The listing builds one solid part. Answer for the finished solid, in the listing's coordinates (mm). Give positions to 0.01 mm unless a question says otherwise; leave off trailing zeros. Order: outer loops, then holes, each group sorted by start corner. A loop starts at its lowest first (then second) coordinate and runs counter-clockwise, first axis right, second up. Notation, with made-up numbers: (25.25, -14) - (56.25, -14) arc R13 cw to (56.25, 8) - close; hole circle Ø10 at (-18, 22). An arc over 180 degrees is marked (long way). Use CSV: the item, a comma, the result in double quotes.
```python
from build123d import *

# Parameters (mm, degrees)
F0_W     = 178
F0_H     = 132
F0_R     = 1.6
F0_R_2   = 1.85
F0_R_3   = 4
F1_DEPTH = 25


with BuildPart() as f1:
    # F0 (on Front) → F1 (new body)
    with BuildSketch(Plane.XZ):
        with Locations((0, -66)):
            Rectangle(F0_W, F0_H)
        with Locations((-33, -112)):
            Circle(F0_R, mode=Mode.SUBTRACT)
        with Locations((-78.656854, -85.656854)):
            Circle(F0_R_2, mode=Mode.SUBTRACT)
        with Locations((-73, -88)):
            Circle(F0_R_2, mode=Mode.SUBTRACT)
        with Locations((-67.343146, -85.656854)):
            Circle(F0_R_2, mode=Mode.SUBTRACT)
        with Locations((-81, -80)):
            Circle(F0_R_2, mode=Mode.SUBTRACT)
        with Locations((-78.656854, -74.343146)):
            Circle(F0_R_2, mode=Mode.SUBTRACT)
        with Locations((-73, -80)):
            Circle(F0_R_3, mode=Mode.SUBTRACT)
        with Locations((-67.343146, -74.343146)):
            Circle(F0_R_2, mode=Mode.SUBTRACT)
        with Locations((-73, -72)):
            Circle(F0_R_2, mode=Mode.SUBTRACT)
        with Locations((-65, -80)):
            Circle(F0_R_2, mode=Mode.SUBTRACT)
        with Locations((19.5, -108)):
            Circle(F0_R, mode=Mode.SUBTRACT)
        with Locations((19.5, -80)):
            Circle(F0_R, mode=Mode.SUBTRACT)
        with Locations((65.343146, -85.656854)):
            Circle(F0_R_2, mode=Mode.SUBTRACT)
        with Locations((71, -88)):
            Circle(F0_R_2, mode=Mode.SUBTRACT)
        with Locations((76.656854, -85.656854)):
            Circle(F0_R_2, mode=Mode.SUBTRACT)
        with Locations((63, -80)):
            Circle(F0_R_2, mode=Mode.SUBTRACT)
        with Locations((65.343146, -74.343146)):
            Circle(F0_R_2, mode=Mode.SUBTRACT)
        with Locations((71, -80)):
            Circle(F0_R_3, mode=Mode.SUBTRACT)
        with Locations((76.656854, -74.343146)):
            Circle(F0_R_2, mode=Mode.SUBTRACT)
        with Locations((79, -80)):
            Circle(F0_R_2, mode=Mode.SUBTRACT)
        with Locations((71, -72)):
            Circle(F0_R_2, mode=Mode.SUBTRACT)
        with Locations((-33, -64)):
            Circle(F0_R, mode=Mode.SUBTRACT)
        with Locations((-33, -36)):
            Circle(F0_R_2, mode=Mode.SUBTRACT)
        with Locations((-78.656854, -21.656854)):
            Circle(F0_R_2, mode=Mode.SUBTRACT)
        with Locations((-73, -24)):
            Circle(F0_R_2, mode=Mode.SUBTRACT)
        with Locations((-67.343146, -21.656854)):
            Circle(F0_R_2, mode=Mode.SUBTRACT)
        with Locations((-81, -16)):
            Circle(F0_R_2, mode=Mode.SUBTRACT)
        with Locations((-78.656854, -10.343146)):
            Circle(F0_R_2, mode=Mode.SUBTRACT)
        with Locations((-73, -16)):
            Circle(F0_R_3, mode=Mode.SUBTRACT)
        with Locations((-67.343146, -10.343146)):
            Circle(F0_R_2, mode=Mode.SUBTRACT)
        with Locations((-73, -8)):
            Circle(F0_R_2, mode=Mode.SUBTRACT)
        with Locations((-65, -16)):
            Circle(F0_R_2, mode=Mode.SUBTRACT)
        with Locations((-33, -6)):
            Circle(F0_R_2, mode=Mode.SUBTRACT)
        with Locations((39, -36)):
            Circle(F0_R_2, mode=Mode.SUBTRACT)
        with Locations((39, -6)):
            Circle(F0_R_2, mode=Mode.SUBTRACT)
        with Locations((65.343146, -21.656854)):
            Circle(F0_R_2, mode=Mode.SUBTRACT)
        with Locations((71, -24)):
            Circle(F0_R_2, mode=Mode.SUBTRACT)
        with Locations((76.656854, -21.656854)):
            Circle(F0_R_2, mode=Mode.SUBTRACT)
        with Locations((63, -16)):
            Circle(F0_R_2, mode=Mode.SUBTRACT)
        with Locations((65.343146, -10.343146)):
            Circle(F0_R_2, mode=Mode.SUBTRACT)
        with Locations((71, -16)):
            Circle(F0_R_3, mode=Mode.SUBTRACT)
        with Locations((76.656854, -10.343146)):
            Circle(F0_R_2, mode=Mode.SUBTRACT)
        with Locations((79, -16)):
            Circle(F0_R_2, mode=Mode.SUBTRACT)
        with Locations((71, -8)):
            Circle(F0_R_2, mode=Mode.SUBTRACT)
    extrude(amount=F1_DEPTH)


solid = f1.part
```
Item 1: The part is cut by section A-A (z = -16). Give the vertices of the cut face in (x, y), and give its area (3 significant figures).
Taken from the geometry:
outline,"(-89, -25) - (-82.85, -25) - (-82.85, 0) - (-89, 0) - close; (-79.15, -25) - (-77, -25) - (-77, 0) - (-79.15, 0) - close; (-69, -25) - (-66.85, -25) - (-66.85, 0) - (-69, 0) - close; (-63.15, -25) - (61.15, -25) - (61.15, 0) - (-63.15, 0) - close; (64.85, -25) - (67, -25) - (67, 0) - (64.85, 0) - close; (75, -25) - (77.15, -25) - (77.15, 0) - (75, 0) - close; (80.85, -25) - (89, -25) - (89, 0) - (80.85, 0) - close"
area,"3,680 mm^2"
Item 2: The part is cut by section B-B (y = -19.5). Count the separate pieces of the cut face and the enclosed holes in it, and give its area (3 significant figures).
Taken from the geometry:
separate pieces,"1"
enclosed holes,"44"
area,"22,900 mm^2"
Item 3: This flat-tipped pin is pushed along its axis until it touches: pin 1 (6 mm diameter, centred on x = 65.34, z = -21.66, fed in from +Y). Where does it stop, or does it pass through?
Taken from the geometry:
pin 1,"y = 0"
Item 4: The mould has two halves that part along Z. Classify faces 1 (the face through (-1, -12, -132)), 2 (the face through (-1, -25, -65)), 3 (the face through (-79.235, -12.325, -15.444)): +Z half, -Z half, draft (parallel to the pull), parting line (faces both ways), or undercut.
Taken from the geometry:
face 1,"-Z half"
face 2,"draft"
face 3,"undercut"
Item 5: Find the intervals of material crossed by line 1 along Z through (x, y) = (-81, -16.75); line 2 along X through (y, z) = (-14.5, -88); line 3 along Z through (x, y) = (68.5, -5.75), in increasing order.
Taken from the geometry:
line 1,"-132 to -81.85, -78.15 to -17.85, -14.15 to 0"
line 2,"-89 to -74.85, -71.15 to 69.15, 72.85 to 89"
line 3,"-132 to -83.12, -76.88 to -19.12, -12.88 to 0"
